Part model, mm, in its own coordinate system. Give positions to 0.01 mm unless a question says otherwise; leave off trailing zeros. Write each loop counter-clockwise with the first axis right and the second up, starting at its lowest first coordinate (ties: lowest second). Pieces come first, ordered by that corner, then holes. Notation, with made-up numbers: (29.25, 55) - (55.25, 55) arc R23 cw to (55.25, 81) - close; hole circle Ø2 at (-12, 52). An arc over 180 degrees is marked (long way). Answer in a Markdown table with one row per item. Add a question column.
1. Band-saw the part on A-A on y = -19.75. Write the cut outline in (x, z), plus the area to 3 significant figures.
2. Probe line 1 along Y through (x, z) = (9.25, -6.15); line 2 along X through (y, z) = (-16.25, -6.2); line 3 along X through (y, z) = (-30.5, -5.45). List the from-to ranges inside material, lowest first.
3. Band-saw the part on B-B on x = 11.5. Write the cut outline in (y, z).
4. Band-saw the part on C-C on z = -5.7. Write the cut outline in (x, y), plus the area to 3 significant figures.
Autodesk Inventor part; units mm, degrees
ref_plane "Work Plane1" through (-8, -18, 2.25) normal (0, 0, 1) x (1, 0, 0)
ref_plane "YZ Plane" through (0, 0, 0) normal (1, 0, 0) x (0, 1, 0)
ref_plane "XZ Plane" through (0, 0, 0) normal (0, 1, 0) x (-1, 0, 0)
ref_plane "Work Plane1" through (-8, -18, 2.25) normal (0, 0, 1) x (1, 0, 0)
ref_plane "Work Plane2" through (16.1776, -21.6969, -6.3588) normal (0, 0, 1) x (1, 0, 0)
sketch "Sketch6" plane through (16.1776, -21.6969, -6.3588) normal (0, 0, 1) x (1, 0, 0)
  circle A0 centre (6.9, -9.5) radius 1.2
  circle A1 centre (-6.9, -6.4) radius 1.2
  circle A2 centre (6.9, 6.4) radius 1.2
  circle A3 centre (-7.9, 7.4) radius 0.4
  line L0 (4.2, -7) -> (-1.2, -7)
  arc A4 (-8.5, 0.3) -> (-1.2, -7) centre (-1.2, 0.3) ccw
  line L1 (-8.5, 0.3) -> (-8.5, 2.7)
  arc A5 (-4.2, 7) -> (-8.5, 2.7) centre (-4.2, 2.7) ccw
  line L2 (-4.2, 7) -> (1.2, 7)
  arc A6 (8.5, -0.3) -> (1.2, 7) centre (1.2, -0.3) ccw
  line L3 (8.5, -0.3) -> (8.5, -2.7)
  arc A7 (4.2, -7) -> (8.5, -2.7) centre (4.2, -2.7) ccw
  line L4 (-4.2738, -7.5) -> (-4.2738, -24.5)
  line L5 (-4.2738, -7.5) -> (4.2738, -7.5)
  line L6 (4.2738, -24.5) -> (4.2738, -7.5)
  line L7 (9, -24.5) -> (4.2738, -24.5)
  line L8 (9, -24.5) -> (9, 8.5)
  line L9 (9, 8.5) -> (-9, 8.5)
  line L10 (-9, 8.5) -> (-9, -24.5)
  line L11 (-4.2738, -24.5) -> (-9, -24.5)
  line L12 (1.2, 6.2) -> (-4.2, 6.2)
  arc A8 (-4.2, 6.2) -> (-7.7, 2.7) centre (-4.2, 2.7) ccw
  line L13 (-7.7, 2.7) -> (-7.7, 0.3)
  arc A9 (-7.7, 0.3) -> (-1.2, -6.2) centre (-1.2, 0.3) ccw
  line L14 (-1.2, -6.2) -> (4.2, -6.2)
  arc A10 (4.2, -6.2) -> (7.7, -2.7) centre (4.2, -2.7) ccw
  line L15 (7.7, -2.7) -> (7.7, -0.3)
  arc A11 (7.7, -0.3) -> (1.2, 6.2) centre (1.2, -0.3) ccw
  line L16 (-7.2, 0.3) -> (-7.2, 2.7)
  arc A12 (-4.2, 5.7) -> (-7.2, 2.7) centre (-4.2, 2.7) ccw
  line L17 (-4.2, 5.7) -> (1.2, 5.7)
  arc A13 (7.2, -0.3) -> (1.2, 5.7) centre (1.2, -0.3) ccw
  line L18 (7.2, -0.3) -> (7.2, -2.7)
  arc A14 (4.2, -5.7) -> (7.2, -2.7) centre (4.2, -2.7) ccw
  line L19 (4.2, -5.7) -> (-1.2, -5.7)
  arc A15 (-7.2, 0.3) -> (-1.2, -5.7) centre (-1.2, 0.3) ccw
  line L20 (8.5, -0.3) -> (8.5, -2.7)
  arc A16 (8.5, -0.3) -> (1.2, 7) centre (1.2, -0.3) ccw
  line L21 (-4.2, 7) -> (1.2, 7)
  arc A17 (-4.2, 7) -> (-8.5, 2.7) centre (-4.2, 2.7) ccw
  line L22 (-8.5, 0.3) -> (-8.5, 2.7)
  arc A18 (-8.5, 0.3) -> (-1.2, -7) centre (-1.2, 0.3) ccw
  line L23 (4.2, -7) -> (-1.2, -7)
  arc A19 (4.2, -7) -> (8.5, -2.7) centre (4.2, -2.7) ccw
  arc A20 (-4.2, 6.2) -> (-7.7, 2.7) centre (-4.2, 2.7) ccw
  line L24 (1.2, 6.2) -> (-4.2, 6.2)
  arc A21 (7.7, -0.3) -> (1.2, 6.2) centre (1.2, -0.3) ccw
  line L25 (7.7, -2.7) -> (7.7, -0.3)
  arc A22 (4.2, -6.2) -> (7.7, -2.7) centre (4.2, -2.7) ccw
  line L26 (-1.2, -6.2) -> (4.2, -6.2)
  arc A23 (-7.7, 0.3) -> (-1.2, -6.2) centre (-1.2, 0.3) ccw
  line L27 (-7.7, 2.7) -> (-7.7, 0.3)
  line L28 (-1.4516, 1.7) -> (-0.5158, 1.7)
  arc A24 (2.07, 0.2211) -> (-0.5158, 1.7) centre (-0.5158, -1.3) ccw
  line L29 (2.07, 0.2211) -> (2.3135, -0.193)
  arc A25 (1.4516, -1.7) -> (2.3135, -0.193) centre (1.4516, -0.7) ccw
  line L30 (1.4516, -1.7) -> (0.5158, -1.7)
  arc A26 (-2.07, -0.2211) -> (0.5158, -1.7) centre (0.5158, 1.3) ccw
  line L31 (-2.07, -0.2211) -> (-2.3135, 0.193)
  arc A27 (-1.4516, 1.7) -> (-2.3135, 0.193) centre (-1.4516, 0.7) ccw
  arc A28 (-7.2, 0.3) -> (-1.2, -5.7) centre (-1.2, 0.3) ccw
  line L32 (-1.2, -5.7) -> (4.2, -5.7)
  arc A29 (4.2, -5.7) -> (7.2, -2.7) centre (4.2, -2.7) ccw
  line L33 (7.2, -2.7) -> (7.2, -0.3)
  arc A30 (7.2, -0.3) -> (1.2, 5.7) centre (1.2, -0.3) ccw
  line L34 (1.2, 5.7) -> (-4.2, 5.7)
  arc A31 (-4.2, 5.7) -> (-7.2, 2.7) centre (-4.2, 2.7) ccw
  line L35 (-7.2, 2.7) -> (-7.2, 0.3)
  line L36 (-9, 8.5) -> (9, 8.5)
  line L37 (9, 8.5) -> (9, -11.5)
  line L38 (9, -11.5) -> (-9, -11.5)
  line L39 (-9, -11.5) -> (-9, 8.5)
  circle A32 centre (-6.9, -6.4) radius 1.05
  circle A33 centre (6.9, -9.5) radius 1.05
  circle A34 centre (6.9, 6.4) radius 1.05
  circle A35 centre (-7.9, 7.4) radius 0.6
  circle A36 centre (-7.9, 7.4) radius 2.25
  line L40 (-4.2, 2.7) -> (4.2, -2.7)
  line L41 (-4.2, 2.7) -> (-5.0412, 3.2408)
  line L42 (4.2, -2.7) -> (5.0412, -3.2408)
  circle A37 centre (-5.0412, 3.2408) radius 2.5
  circle A38 centre (5.0412, -3.2408) radius 2.5
  point P0 (-16.1776, 21.6969)
  point P1 (-9, -11.5)
  dimension "d36" = 20
  dimension "d37" = 2.1
  dimension "d38" = 2.1
  dimension "d39" = 2.1
  dimension "d40" = 1.2
  dimension "d41" = 4.5
  dimension "d42" = 1
  dimension "d43" = 1
  dimension "d44" = 5
  dimension "d45" = 5
extrude "Extrusion4" add sketch "Sketch6" along normal blind 3 contours A0 | A1 | A2 | A7 L3 A6 L2 A5 A36 L9 L8 L38 L6 L5 L4 L10 L1 A4 L0 | L0 A4 L1 A5 A36 L2 A6 L3 A7 | A36 L10 L9 A5 | A5 A36 | L4 L5 L6 L38 | A11 L15 A10 A38 L18 A13 L17 A12 A37 A8 L12 | A37 L16 A15 L19 A14 A38 A10 L14 A9 L13 A8 | A12 L17 A13 L18 A38 L40 A25 L29 A24 L28 A27 A37 | A37 L40 A27 L31 A26 L30 A25 A38 A14 L19 A15 L16 | L40 A25 L30 A26 L31 A27 | A27 L28 A24 L29 A25 L40
move faces "Move2" translate (0, 0, -2) faces at (13.0665, -31.2809, -3.3588)
properties part number "water line connector"
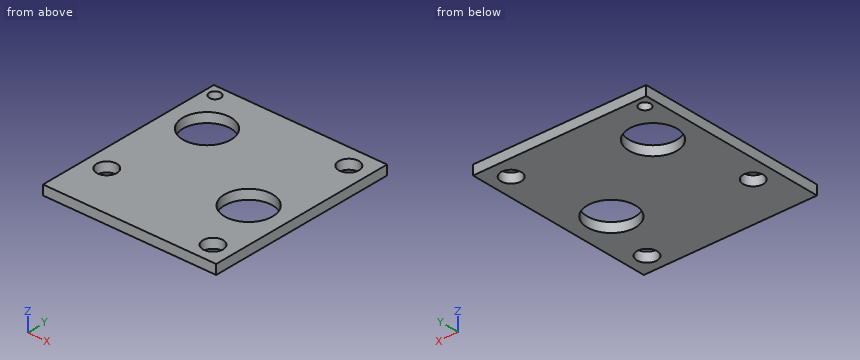
Values:
| question | item | result |
|---|---|---|
| 1 | outline | (7.18, -6.36) - (9, -6.36) - (9, -5.36) - (7.18, -5.36) - close; (13.28, -6.36) - (25.18, -6.36) - (25.18, -5.36) - (13.28, -5.36) - close |
| 1 | area | 13.7 mm² |
| 2 | line 1 | y = -33.2 to -29.15, -27.05 to -20.1, -16.82 to -13.2 |
| 2 | line 2 | x = 7.18 to 9.96, 12.31 to 22.64, 23.52 to 25.18 |
| 2 | line 3 | x = 7.18 to 22.29, 23.86 to 25.18 |
| 3 | outline | (-33.2, -6.36) - (-20.93, -6.36) - (-20.93, -5.36) - (-33.2, -5.36) - close; (-15.98, -6.36) - (-13.2, -6.36) - (-13.2, -5.36) - (-15.98, -5.36) - close |
| 4 | outline | (7.18, -33.2) - (25.18, -33.2) - (25.18, -13.2) - (7.18, -13.2) - close; hole circle Ø1.2 at (8.28, -14.3); hole circle Ø2.1 at (9.28, -28.1); hole circle Ø5 at (11.14, -18.46); hole circle Ø5 at (21.22, -24.94); hole circle Ø2.1 at (23.08, -31.2); hole circle Ø2.1 at (23.08, -15.3) |
| 4 | area | 309 mm² |
